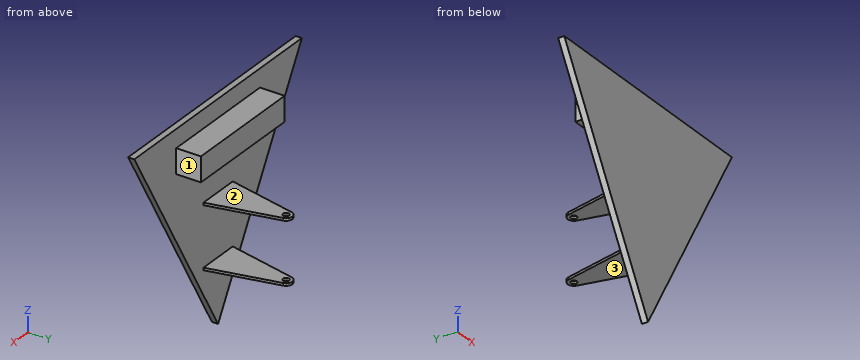
```python
from build123d import *

# Parameters (mm, degrees)
BOSS_EXTRUDE1_DEPTH = 5
SKETCH2_W           = 35
SKETCH2_H           = 2
BOSS_EXTRUDE2_DEPTH = 60
CUT_EXTRUDE1_DEPTH  = 60
SKETCH4_R           = 2.5
CUT_EXTRUDE2_DEPTH  = 60
SKETCH5_W           = 100
SKETCH5_H           = 20
BOSS_EXTRUDE3_DEPTH = 20


with BuildPart() as part:
    # Sketch1 → Boss-Extrude1 (new body)
    with BuildSketch(Plane(origin=(0, 0, 0), x_dir=(1, 0, 0), z_dir=(0, 1, 0))):
        Polygon((0, 115.470053838), (-100, -57.735026919), (100, -57.735026919), align=None)
    extrude(amount=BOSS_EXTRUDE1_DEPTH)

    # Sketch2 → Boss-Extrude2 (add)
    with BuildSketch(Plane(origin=(0, 5, 0), x_dir=(1, 0, 0), z_dir=(0, 1, 0))):
        with Locations((0, 65)):
            Rectangle(SKETCH2_W, SKETCH2_H)
        with Locations((0, 15)):
            Rectangle(SKETCH2_W, SKETCH2_H)
    extrude(amount=BOSS_EXTRUDE2_DEPTH)

    # Sketch3 → Cut-Extrude1 (cut)
    with BuildSketch(Plane.XY.offset(-14)):
        with BuildLine():
            Line((-17.5, 65), (-17.5, 5))
            Line((-17.5, 5), (-4.898590768, 61.001902433))
            ThreePointArc((-4.898590768, 61.001902433), (-4.878030477, 61.097642323), (-4.855599196, 61.192961208))
            ThreePointArc((-4.855599196, 61.192961208), (-3.085060288, 63.934768484), (0, 65))
            Line((0, 65), (-17.5, 65))
        make_face()
        with BuildLine():
            Line((17.5, 65), (0, 65))
            ThreePointArc((0, 65), (3.085060288, 63.934768484), (4.855599196, 61.192961208))
            ThreePointArc((4.855599196, 61.192961208), (4.878030477, 61.097642323), (4.898590768, 61.001902433))
            Line((4.898590768, 61.001902433), (17.5, 5))
            Line((17.5, 5), (17.5, 65))
        make_face()
    extrude(amount=-CUT_EXTRUDE1_DEPTH, mode=Mode.SUBTRACT)

    # Sketch4 → Cut-Extrude2 (cut)
    with BuildSketch(Plane.XY.offset(-14)):
        with Locations((0, 60)):
            Circle(SKETCH4_R)
    extrude(amount=-CUT_EXTRUDE2_DEPTH, mode=Mode.SUBTRACT)

    # Sketch5 → Boss-Extrude3 (add)
    with BuildSketch(Plane(origin=(0, 5, 0), x_dir=(1, 0, 0), z_dir=(0, 1, 0))):
        with Locations((0, -33)):
            Rectangle(SKETCH5_W, SKETCH5_H)
    extrude(amount=BOSS_EXTRUDE3_DEPTH)


solid = part.part
```
Input: part model. Units: mm. Frame: model coordinates. Face numbers are marked on the shaded views. A direction names the side the tool comes from. Give positions to 0.01 mm unless a question says otherwise; leave off trailing zeros. Loops run counter-clockwise (first coordinate to the right, second up) from the corner with the lowest first, then second, coordinate; pieces in that order, holes last.
1) Section query C-C on x = 10. Return the cut outline in (y, z).
A:
outline: (0, -98.15) - (5, -98.15) - (5, -66) - (38.33, -66) - (38.33, -64) - (5, -64) - (5, -16) - (38.33, -16) - (38.33, -14) - (5, -14) - (5, 23) - (25, 23) - (25, 43) - (5, 43) - (5, 57.74) - (0, 57.74) - close
2) Section query A-A on z = 36.5. Return the cut outline in (x, y).
A:
outline: (-87.74, 0) - (87.74, 0) - (87.74, 5) - (50, 5) - (50, 25) - (-50, 25) - (-50, 5) - (-87.74, 5) - close
3) Line query: L1, parallel to Z at x = 12, y = 23.5; L2, parallel to Y at x = 23, z = 34.5; L3, parallel to Z at x = -5.5, y = 53.5. Output: solid intervals per line, ascending.
A:
L1: z = -66 to -64, -16 to -14, 23 to 43
L2: y = 0 to 25
L3: z = -66 to -64, -16 to -14
4) Contact query for flat-ended pins moving along their axis: pin 1 (16 mm diameter, centred on x = -5, y = 17.5, fed in from +Z); pin 2 (4 mm diameter, centred on x = 0, y = 60, fed in from +Z); pin 3 (6 mm diameter, centred on x = 7.5, y = 12.5, fed in from -Z); pin 4 (5 mm diameter, centred on x = -39.5, z = -46, fed in from -Y). Output: stop coordinate, or through.
A:
pin 1: stops at z = 43
pin 2: passes through
pin 3: stops at z = -66
pin 4: stops at y = 0
5) Section query B-B on x = 45. Return the cut outline in (y, z), and give its area (3 significant figures).
A:
outline: (0, -37.53) - (5, -37.53) - (5, 23) - (25, 23) - (25, 43) - (5, 43) - (5, 57.74) - (0, 57.74) - close
area: 876 mm2
6) Section query D-D on z = -48. Return the cut outline in (x, y).
A:
outline: (-38.95, 0) - (38.95, 0) - (38.95, 5) - (-38.95, 5) - close
7) Reachability of the marked faces 1, 2 and 3 from +Z, -Z, +X, -X, +Y, -Y: full face, straight path, thin tool, end or side. Return the list, or none.
A:
face 1: +Z, -Z, +X, +Y
face 2: +X, -X, +Y
face 3: -Z, +X, -X, +Y
